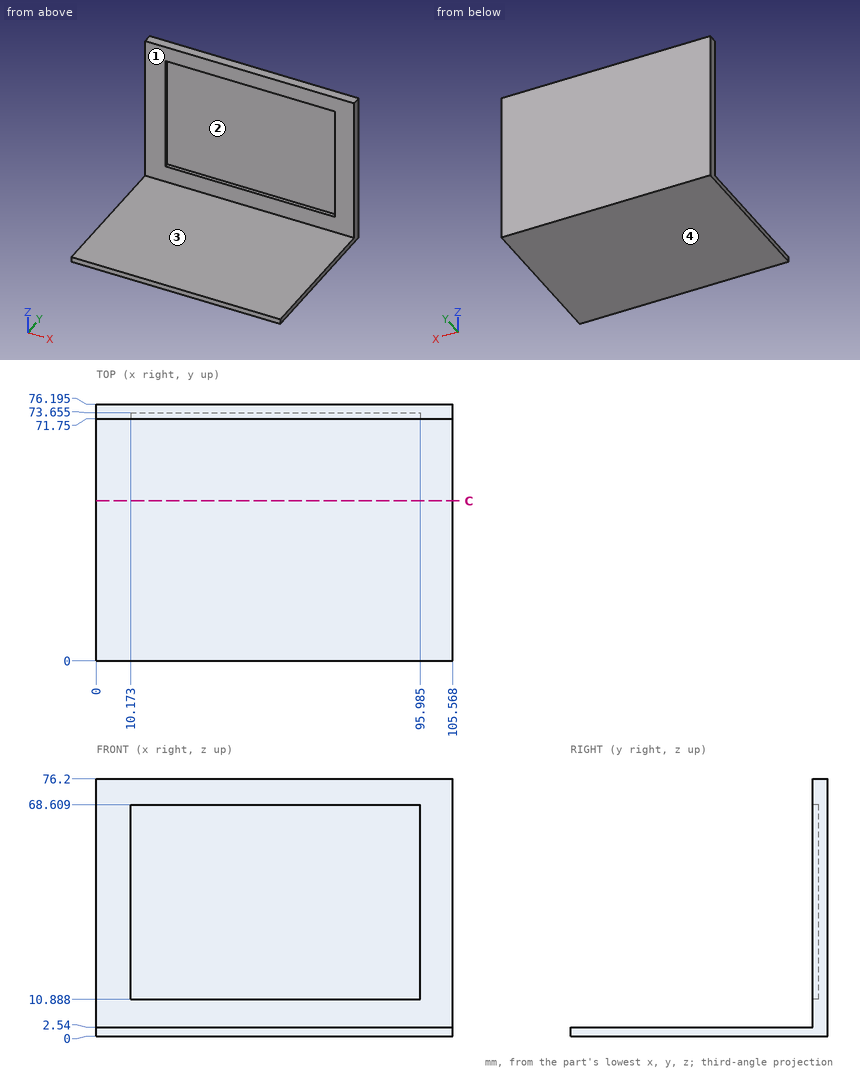
The drawing under review shows one solid part. Ordinate dimensions are in mm from its lowest x, y, z. Round coordinates to 2 decimals unless told otherwise and drop trailing zeros. Write each loop counter-clockwise with the first axis right and the second up, starting at its lowest first coordinate (ties: lowest second). Pieces come first, ordered by that corner, then holes. Notation, with made-up numbers: (-28.5, -1.5) - (16.5, -1.5) arc R6 cw to (16.5, 9.5) - close; hole circle Ø2 at (65, 74). An arc over 180 degrees is marked (long way). Use a Markdown table: item, result. Add a question column.
1. Mouldability with a two-part tool opening along Z and no side actions: class the marked faces 1, 2, 3 and 4 as +Z half, -Z half, draft (parallel to the pull), parting line (faces both ways), or undercut.
2. Wall thickness on probe 1 along Z at (x, y) = (49, 53); probe 2 along Y at (x, z) = (41, 25) (1 decimal): over which ranges is each line inside the solid? List them lowest first.
3. Clearance check with flat-ended pins moving along their axes: pin 1 (0.6 mm diameter, centred on x = 74, y = 72.5, fed in from -Z); pin 2 (10 mm diameter, centred on x = 68.5, z = 18, fed in from -Y) (1 decimal). State where each tip first meets the part, or that it passes through.
4. We need section C-C (y = 47.5). State the section outline as (x, z) points, then the cut area to 3 significant figures.
Output:
| question | item | result |
|---|---|---|
| 1 | face 1 | draft |
| 1 | face 2 | undercut |
| 1 | face 3 | +Z half |
| 1 | face 4 | -Z half |
| 2 | probe 1 | z = 0 to 2.54 |
| 2 | probe 2 | y = 73.7 to 76.2 |
| 3 | pin 1 | stops at z = 0 |
| 3 | pin 2 | stops at y = 73.7 |
| 4 | outline | (0, 0) - (105.57, 0) - (105.57, 2.54) - (0, 2.54) - close |
| 4 | area | 268 mm2 |
